Build history of the part. All positions in model axes, mm. Face numbers are marked on the shaded views. Give positions to 0.01 mm unless a question says otherwise; leave off trailing zeros. Write each loop counter-clockwise with the first axis right and the second up, starting at its lowest first coordinate (ties: lowest second). Pieces come first, ordered by that corner, then holes. Notation, with made-up numbers: M -39,69.5 L -24,69.5 A22 ccw -24,107.5 Z; hole C 13.25,3.5 d7. An arc over 180 degrees is marked long. Return JSON: item names as keys, results as strings. Group by question number.
Q1. Pull direction X, two halves, no side cores. Call the marked faces 1, 2 and 3: +X half, -X half, draft (parallel to the pull), parting line (faces both ways), or undercut.
Q2. Band-saw the part on C-C, the plane y = -26.5. Give the cut face in (x, z).
Q3. Band-saw the part on D-D, the plane x = 21.5. Give the cut face in (y, z), then the cut area to 3 significant figures.
Q4. Band-saw the part on B-B, the plane x = -5. Give the cut face in (y, z).
Q5. Band-saw the part on A-A, the plane y = 13.5. Give the cut face in (x, z).
Q6. Wall check: probe 1 along Y at (x, z) = (21.5, 3.2); probe 2 along Y at (x, z) = (-31.5, 4.9); probe 3 along X at (y, z) = (3.5, 7.5). Give the ranges that are in metal, low to high.
Q7. Flat gauge pins, fed straight in: pin 1 Ø1.6 at (x, y) = (-31.5, 26.5) entering from +Z; pin 2 Ø2.5 at (x, y) = (31.5, -26.5) entering from +Z; pin 3 Ø2 at (x, y) = (12.5, -30.5) entering from +Z. Where does each tip first touch, or does it go through?
from build123d import *

# Parameters (mm, degrees)
F3_W      = 73
F3_H      = 63
F3_W_2    = 69
F3_H_2    = 59
F4_DEPTH  = 9.5
F5_DEPTH  = 2
F6_W      = 6
F6_H      = 6
F6_R      = 1
F7_DEPTH  = 4
F8_W      = 26.5
F8_H      = 2
F9_DEPTH  = 2
F10_W     = 26.5
F10_H     = 2
F10_W_2   = 17.5
F11_DEPTH = 2


with BuildPart() as f4:
    # F3 (on Top) → F4 (new body)
    with BuildSketch(Plane.XY):
        Rectangle(F3_W, F3_H)
        Rectangle(F3_W_2, F3_H_2, mode=Mode.SUBTRACT)
    extrude(amount=F4_DEPTH)

    # F3 (on Top) → F5 (join)
    with BuildSketch(Plane.XY):
        Rectangle(F3_W_2, F3_H_2)
    extrude(amount=F5_DEPTH)

    # F6 (on face) → F7 (join)
    with BuildSketch(Plane.XY.offset(2)):
        with Locations((21.5, 13.5)):
            Rectangle(F6_W, F6_H)
        with Locations((21.5, 13.5)):
            Circle(F6_R, mode=Mode.SUBTRACT)
        with Locations((31.5, -26.5)):
            Rectangle(F6_W, F6_H)
        with Locations((31.5, -26.5)):
            Circle(F6_R, mode=Mode.SUBTRACT)
        with Locations((-31.5, 26.5)):
            Rectangle(F6_W, F6_H)
        with Locations((-31.5, 26.5)):
            Circle(F6_R, mode=Mode.SUBTRACT)
        with Locations((-31.5, -26.5)):
            Rectangle(F6_W, F6_H)
        with Locations((-31.5, -26.5)):
            Circle(F6_R, mode=Mode.SUBTRACT)
    extrude(amount=F7_DEPTH)

    # F8 (on face) → F9 (cut, through all)
    with BuildSketch(Plane.XZ.offset(31.5)):
        with Locations((15.25, 8.5)):
            Rectangle(F8_W, F8_H)
        with Locations((-15.25, 8.5)):
            Rectangle(F8_W, F8_H)
    extrude(amount=-F9_DEPTH, mode=Mode.SUBTRACT)

    # F10 (on face) → F11 (cut, through all)
    with BuildSketch(Plane(origin=(-36.5, 0, 0), x_dir=(0, -1, 0), z_dir=(-1, 0, 0))):
        with Locations((10.25, 8.5)):
            Rectangle(F10_W, F10_H)
        with Locations((-14.75, 8.5)):
            Rectangle(F10_W_2, F10_H)
    extrude(amount=-F11_DEPTH, mode=Mode.SUBTRACT)


solid = f4.part
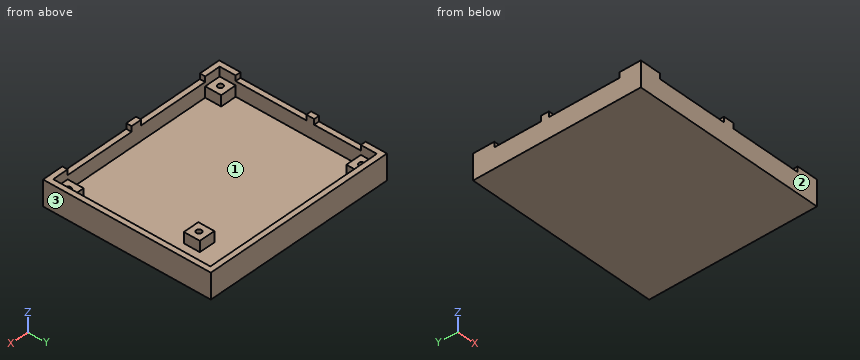
From the geometry:
{
 "1": {"face 1": "undercut", "face 2": "draft", "face 3": "+X half"},
 "2": {"outline": "M -36.5,0 L 36.5,0 L 36.5,9.5 L 34.5,9.5 L 34.5,6 L 32.5,6 L 32.5,2 L 30.5,2 L 30.5,6 L 28.5,6 L 28.5,2 L -28.5,2 L -28.5,6 L -30.5,6 L -30.5,2 L -32.5,2 L -32.5,6 L -34.5,6 L -34.5,9.5 L -36.5,9.5 Z"},
 "3": {"outline": "M -31.5,0 L 31.5,0 L 31.5,9.5 L 29.5,9.5 L 29.5,2 L 16.5,2 L 16.5,6 L 14.5,6 L 14.5,2 L 12.5,2 L 12.5,6 L 10.5,6 L 10.5,2 L -29.5,2 L -29.5,7.5 L -31.5,7.5 Z", "area": "168 mm^2"},
 "4": {"outline": "M -31.5,0 L 31.5,0 L 31.5,9.5 L 29.5,9.5 L 29.5,2 L -29.5,2 L -29.5,7.5 L -31.5,7.5 Z"},
 "5": {"outline": "M -36.5,0 L 36.5,0 L 36.5,9.5 L 34.5,9.5 L 34.5,2 L 24.5,2 L 24.5,6 L 22.5,6 L 22.5,2 L 20.5,2 L 20.5,6 L 18.5,6 L 18.5,2 L -34.5,2 L -34.5,7.5 L -36.5,7.5 Z"},
 "6": {"probe 1": "y = -31.5 to -29.5, 10.5 to 12.5, 14.5 to 16.5, 29.5 to 31.5", "probe 2": "y = -31.5 to -27.5, -25.5 to -23.5, 23.5 to 25.5, 27.5 to 31.5", "probe 3": "x = -36.5 to -34.5, 34.5 to 36.5"},
 "7": {"pin 1": "stops at z = 2", "pin 2": "stops at z = 6", "pin 3": "stops at z = 7.5"}
}
